For this review, take the finished solid that the model builds, in its own axes (mm). A direction names the side the tool comes from. Give positions to 0.01 mm unless a question says otherwise; leave off trailing zeros. Order: outer loops, then holes, each group sorted by start corner. A loop starts at its lowest first (then second) coordinate and runs counter-clockwise, first axis right, second up.
Item 1: The part is to be moulded in two halves that separate along Z. For faces 4 (the flat face through (22, -9, 5)), 5 (the cylindrical face through (2.3, 6.6, -4.2)), 6 (the cylindrical face through (12.09, 7.45, 9.71)), say which applies: released by +Z, released by -Z, zero draft, split by the parting line, or undercut.
Item 2: Consider section B-B (x = 20.5). Give the boundary of the cut face in (y, z), plus the area to 3 significant figures.
Item 3: Consider section A-A (x = 3). Give the boundary of the cut face in (y, z) (3 decimals).
Item 4: Machinability: for faces 1 (the cylindrical face through (20.08, 3.25, -10.31)), 2 (the flat face through (0, -8, 1)), 3 (the cylindrical face through (3.204, -5.37, 7.003)), which of the approach directions +Z, -Z, +X, -X, +Y, -Y give a long, thin tool a straight path to every point of the face, cutting with its end or side? Answer none if there is none.
Item 5: For probe 1 along Y at (x, z) = (3.7, 0) (3 decimals); probe 2 along Y at (x, z) = (18.25, 0); probe 3 along Z at (x, y) = (12.5, 0), list the stretches that pass through material, from the lowest coordinate up.
Item 6: For P1, Ø1, axis at x = 11, y = 6, coming from the +Z side; P2, Ø3, axis at x = 6, y = 7, coming from the -Z side; P3, Ø1.5, axis at x = 2.5, z = 4.5, coming from the -Y side; P4, Ø3, axis at y = 6.5, z = 2.5, coming from the -X side, all flat-tipped, find the tip position at first contact; note any pin that passes through.
```python
from build123d import *

# Parameters (mm, degrees)
SKETCH1_R           = 8.825
SKETCH1_R_2         = 7.825
BOSS_EXTRUDE1_DEPTH = 10
SKETCH2_R           = 12.24
SKETCH2_R_2         = 7.825
BOSS_EXTRUDE2_DEPTH = 12
CHAMFER1_SIZE       = 3.5
SKETCH3_R           = 9.8
CUT_EXTRUDE1_DEPTH  = 12
CHAMFER2_SIZE       = 4
FILLET1_R           = 3
SKETCH4_R           = 12.810143369
SKETCH4_R_2         = 10.810143369
CUT_EXTRUDE2_DEPTH  = 7
CHAMFER3_SIZE       = 2
FILLET2_R           = 3
FILLET3_R           = 3
FILLET4_R           = 0.1


with BuildPart() as part:
    # Sketch1 → Boss-Extrude1 (new body)
    with BuildSketch(Plane(origin=(0, 0, 0), x_dir=(0, 0, -1), z_dir=(1, 0, 0))):
        Circle(SKETCH1_R)
        Circle(SKETCH1_R_2, mode=Mode.SUBTRACT)
    extrude(amount=BOSS_EXTRUDE1_DEPTH)

    # Sketch2 → Boss-Extrude2 (add)
    with BuildSketch(Plane(origin=(10, 0, 0), x_dir=(0, 0, -1), z_dir=(1, 0, 0))):
        Circle(SKETCH2_R)
        Circle(SKETCH2_R_2, mode=Mode.SUBTRACT)
    extrude(amount=BOSS_EXTRUDE2_DEPTH)

    # Chamfer1
    # the kernel refuses this chamfer: 3.5 mm, written as the material it adds along each edge
    with BuildSketch(Plane(origin=(10, 0, 0), x_dir=(0, 0, -1), z_dir=(0, -1, 0))) as chamfer1_piece_1_section:
        Polygon((8.825, -CHAMFER1_SIZE), (8.825 + CHAMFER1_SIZE, 0), (8.825, 0), align=None)
    chamfer1_piece_1 = revolve(axis=Axis((10, 0, 0), (1, 0, 0)), mode=Mode.PRIVATE)
    chamfer1_piece_1 = chamfer1_piece_1 & Plane(origin=(8.210974628, 0, 0), x_dir=(0, 0, -1), z_dir=(-1, 0, 0)) * Cylinder(12.24, 50, mode=Mode.PRIVATE)
    add(chamfer1_piece_1)

    # Sketch3 → Cut-Extrude1 (cut)
    with BuildSketch(Plane(origin=(22, 0, 0), x_dir=(0, 0, -1), z_dir=(1, 0, 0))):
        Circle(SKETCH3_R)
    extrude(amount=-CUT_EXTRUDE1_DEPTH, mode=Mode.SUBTRACT)

    # Chamfer2
    # the kernel refuses this chamfer: 4 mm, written as the material it takes off along each edge
    with BuildSketch(Plane(origin=(10, 0, 0), x_dir=(0, 0, -1), z_dir=(0, 1, 0))) as chamfer2_piece_1_section:
        Polygon((7.825, CHAMFER2_SIZE), (7.825 + CHAMFER2_SIZE, 0), (7.825, 0), align=None)
    chamfer2_piece_1 = revolve(axis=Axis((10, 0, 0), (-1, 0, 0)), mode=Mode.PRIVATE)
    chamfer2_piece_1 = chamfer2_piece_1 & Plane(origin=(6.980894561, 0, 0), x_dir=(0, 0, -1), z_dir=(1, 0, 0)) * Cylinder(9.8, 48, mode=Mode.PRIVATE)
    add(chamfer2_piece_1, mode=Mode.SUBTRACT)

    # Fillet1
    fillet1_edges = [part.edges().sort_by_distance(p)[0] for p in [
        (6, 0, 7.825),
        (7.975, 0, 9.8),
    ]]
    fillet(fillet1_edges, radius=FILLET1_R)

    # Sketch4 → Cut-Extrude2 (cut)
    with BuildSketch(Plane(origin=(22, 0, 0), x_dir=(0, 0, -1), z_dir=(1, 0, 0))):
        Circle(SKETCH4_R)
        Circle(SKETCH4_R_2, mode=Mode.SUBTRACT)
    extrude(amount=-CUT_EXTRUDE2_DEPTH, mode=Mode.SUBTRACT)

    # Chamfer3
    # the kernel refuses this chamfer: 2 mm, written as the material it adds along each edge
    with BuildSketch(Plane(origin=(15, 0, 0), x_dir=(0, 0, -1), z_dir=(0, -1, 0))) as chamfer3_piece_1_section:
        Polygon((10.810143369 + CHAMFER3_SIZE, 0), (10.810143369, CHAMFER3_SIZE), (10.810143369, 0), align=None)
    chamfer3_piece_1 = revolve(axis=Axis((15, 0, 0), (1, 0, 0)), mode=Mode.PRIVATE)
    chamfer3_piece_1 = chamfer3_piece_1 & Plane(origin=(16.276433471, 0, 0), x_dir=(0, 0, -1), z_dir=(-1, 0, 0)) * Cylinder(12.24, 52, mode=Mode.PRIVATE)
    add(chamfer3_piece_1)

    # Fillet2
    fillet2_edges = [part.edges().sort_by_distance(p)[0] for p in [
        (15.570143369, 0, 12.24),
    ]]
    fillet(fillet2_edges, radius=FILLET2_R)

    # Fillet3
    fillet3_edges = [part.edges().sort_by_distance(p)[0] for p in [
        (17, 0, 10.810143369),
    ]]
    fillet(fillet3_edges, radius=FILLET3_R)

    # Fillet4
    fillet4_edges = [part.edges().sort_by_distance(p)[0] for p in [
        (22, 0, 9.8),
        (22, 0, 10.810143369),
    ]]
    fillet(fillet4_edges, radius=FILLET4_R)


solid = part.part
```
Resolved:
1. face 4: zero draft
1. face 5: undercut
1. face 6: split by the parting line
2. outline: circle Ø21.62 at (0, 0); hole circle Ø19.6 at (0, 0)
2. area: 65.4 mm2
3. outline: circle Ø17.65 at (0, 0); hole circle Ø15.65 at (0, 0)
4. face 1: +X
4. face 2: +Z, -Z, -X, +Y, -Y
4. face 3: -X
5. probe 1: y = -8.825 to -7.825, 7.825 to 8.825
5. probe 2: y = -10.81 to -9.8, 9.8 to 10.81
5. probe 3: z = -12.24 to -9.8, 9.8 to 12.24
6. P1: stops at z = 10.93
6. P2: stops at z = -7.32
6. P3: stops at y = -7.99
6. P4: stops at x = 0
